```python
from build123d import *

# Parameters (mm, degrees)
SKETCH1_W                 = 76.2
SKETCH1_H                 = 76.2
BOSS_EXTRUDE1_DEPTH       = 3.175
SKETCH2_W                 = 69.79412
SKETCH2_H                 = 69.79412
BOSS_EXTRUDE2_DEPTH       = 9.525
F_6_32_TAPPED_HOLE1_D     = 2.7051
CIRPATTERN1_COUNT         = 4
SKETCH14_R                = 3.175
CUT_EXTRUDE1_DEPTH        = 56.358016583
SKETCH15_W                = 50.74412
SKETCH15_H                = 26.95956
CUT_EXTRUDE2_DEPTH        = 9.525
FILLET1_R                 = 12.7
F_6_32_TAPPED_HOLE2_D     = 2.7051
F_6_32_TAPPED_HOLE2_DEPTH = 9.652
F_6_32_TAPPED_HOLE2_TIP   = 0.81269403
FILLET1_OF_MIRROR3_R      = 12.7
SKETCH21_W                = 76.2
SKETCH21_H                = 76.2
CUT_EXTRUDE3_DEPTH        = 3.175


with BuildPart() as part:
    # Sketch1 → Boss-Extrude1 (new body)
    with BuildSketch(Plane(origin=(0, 0, 0), x_dir=(1, 0, 0), z_dir=(0, 1, 0))):
        Rectangle(SKETCH1_W, SKETCH1_H)
    extrude(amount=BOSS_EXTRUDE1_DEPTH)

    # Sketch2 → Boss-Extrude2 (add)
    with BuildSketch(Plane(origin=(0, 3.175, 0), x_dir=(1, 0, 0), z_dir=(0, 1, 0))):
        Rectangle(SKETCH2_W, SKETCH2_H)
    extrude(amount=BOSS_EXTRUDE2_DEPTH)

    # Sketch9 → #6-32 Tapped Hole3 (revolve, cut)
    with BuildSketch(Plane(origin=(34.89706, 7.9375, 12.7), x_dir=(0, 0, -1), z_dir=(0, 1, 0))):
        Polygon((0, 0), (0, 11.98869403), (1.35255, 11.176), (1.35255, 0), align=None)
    f_6_32_tapped_hole3 = revolve(axis=Axis((41.24706, 7.9375, 12.7), (-1, 0, 0)), mode=Mode.SUBTRACT)

    # Mirror1: #6-32 Tapped Hole3 across plane
    add(f_6_32_tapped_hole3.mirror(Plane.XY), mode=Mode.SUBTRACT)

    # Mirror2: #6-32 Tapped Hole3 across plane
    add(f_6_32_tapped_hole3.mirror(Plane(origin=(0, 0, 0), x_dir=(0, 0, 1), z_dir=(1, 0, 0))), mode=Mode.SUBTRACT)

    # Mirror2 copy 1 sketch → Mirror2 copy 1 (revolve, cut)
    with BuildSketch(Plane(origin=(-34.89706, 7.9375, -12.7), x_dir=(0, 0, 1), z_dir=(0, 1, 0))):
        Polygon((0, 0), (0, 11.98869403), (1.35255, 11.176), (1.35255, 0), align=None)
    revolve(axis=Axis((-41.24706, 7.9375, -12.7), (1, 0, 0)), mode=Mode.SUBTRACT)

    # #6-32 Tapped Hole1 (through all)
    with Locations(Plane(origin=(0, 0, 0), x_dir=(-1, 0, 0), z_dir=(0, -1, 0))):
        with Locations((-32.5501, 32.5501)):
            f_6_32_tapped_hole1 = Hole(F_6_32_TAPPED_HOLE1_D / 2)

    # CirPattern1: #6-32 Tapped Hole1 ×4 about axis
    cirpattern1_axis = Axis((0, 0, 0), (0, 1, 0))
    for i in range(1, CIRPATTERN1_COUNT):
        add(f_6_32_tapped_hole1.rotate(cirpattern1_axis, i * 360 / CIRPATTERN1_COUNT), mode=Mode.SUBTRACT)

    # Sketch14 → Cut-Extrude1 (cut, through all)
    with BuildSketch(Plane.XZ):
        with Locations(Location((0, 0, 0), (0, 0, 270))):
            Circle(SKETCH14_R)
    extrude(amount=-CUT_EXTRUDE1_DEPTH, mode=Mode.SUBTRACT)

    # Sketch15 → Cut-Extrude2 (cut)
    with BuildSketch(Plane(origin=(0, 12.7, 0), x_dir=(1, 0, 0), z_dir=(0, 1, 0))):
        with Locations((0, -21.41728)):
            Rectangle(SKETCH15_W, SKETCH15_H)
    cut_extrude2 = extrude(amount=-CUT_EXTRUDE2_DEPTH, mode=Mode.SUBTRACT)

    # Fillet1
    # the kernel refuses this fillet: 12.7 mm, written as the material it adds along each edge
    with BuildSketch(Plane(origin=(25.37206, 12.7, 7.9375), x_dir=(0, 0, 1), z_dir=(0, -1, 0))) as fillet1_piece_1_section:
        with BuildLine():
            CenterArc((FILLET1_R, FILLET1_R), FILLET1_R, 180, 90)
            Line((0, FILLET1_R), (0, 0))
            Line((0, 0), (FILLET1_R, 0))
        make_face()
    fillet1_piece_1 = extrude(amount=9.525, mode=Mode.PRIVATE)
    fillet1_piece_1 = fillet1_piece_1 - Plane(origin=(22.423937315, 7.9375, 12.7), x_dir=(0, 0, -1), z_dir=(1, 0, 0)) * Cylinder(1.35255, 70, mode=Mode.PRIVATE)
    add(fillet1_piece_1)
    with BuildSketch(Plane(origin=(-25.37206, 12.7, 7.9375), x_dir=(1, 0, 0), z_dir=(0, -1, 0))) as fillet1_piece_2_section:
        with BuildLine():
            CenterArc((FILLET1_R, FILLET1_R), FILLET1_R, 180, 90)
            Line((0, FILLET1_R), (0, 0))
            Line((0, 0), (FILLET1_R, 0))
        make_face()
    fillet1_piece_2 = extrude(amount=9.525, mode=Mode.PRIVATE)
    fillet1_piece_2 = fillet1_piece_2 - Plane(origin=(-22.423935797, 7.9375, 12.7), x_dir=(0, 0, -1), z_dir=(-1, 0, 0)) * Cylinder(1.35255, 70, mode=Mode.PRIVATE)
    add(fillet1_piece_2)

    # #6-32 Tapped Hole2
    with Locations(Plane.XY.offset(7.9375)):
        with Locations((0, 7.9375)):
            Hole(F_6_32_TAPPED_HOLE2_D / 2, depth=F_6_32_TAPPED_HOLE2_DEPTH)
            with Locations((0, 0, -(F_6_32_TAPPED_HOLE2_DEPTH + F_6_32_TAPPED_HOLE2_TIP / 2))):  # 118° drill point
                Cone(0, F_6_32_TAPPED_HOLE2_D / 2, F_6_32_TAPPED_HOLE2_TIP, mode=Mode.SUBTRACT)

    # Mirror3: Cut-Extrude2 across plane
    add(cut_extrude2.mirror(Plane.XY), mode=Mode.SUBTRACT)

    # Fillet1 of Mirror3
    # the kernel refuses this fillet: 12.7 mm, written as the material it adds along each edge
    with BuildSketch(Plane(origin=(25.37206, 12.7, -7.9375), x_dir=(-1, 0, 0), z_dir=(0, -1, 0))) as fillet1_of_mirror3_piece_1_section:
        with BuildLine():
            CenterArc((FILLET1_OF_MIRROR3_R, FILLET1_OF_MIRROR3_R), FILLET1_OF_MIRROR3_R, 180, 90)
            Line((0, FILLET1_OF_MIRROR3_R), (0, 0))
            Line((0, 0), (FILLET1_OF_MIRROR3_R, 0))
        make_face()
    fillet1_of_mirror3_piece_1 = extrude(amount=9.525, mode=Mode.PRIVATE)
    fillet1_of_mirror3_piece_1 = fillet1_of_mirror3_piece_1 - Plane(origin=(22.423935797, 7.9375, -12.7), x_dir=(0, 0, 1), z_dir=(1, 0, 0)) * Cylinder(1.35255, 70, mode=Mode.PRIVATE)
    add(fillet1_of_mirror3_piece_1)
    with BuildSketch(Plane(origin=(-25.37206, 12.7, -7.9375), x_dir=(0, 0, -1), z_dir=(0, -1, 0))) as fillet1_of_mirror3_piece_2_section:
        with BuildLine():
            CenterArc((FILLET1_OF_MIRROR3_R, FILLET1_OF_MIRROR3_R), FILLET1_OF_MIRROR3_R, 180, 90)
            Line((0, FILLET1_OF_MIRROR3_R), (0, 0))
            Line((0, 0), (FILLET1_OF_MIRROR3_R, 0))
        make_face()
    fillet1_of_mirror3_piece_2 = extrude(amount=9.525, mode=Mode.PRIVATE)
    fillet1_of_mirror3_piece_2 = fillet1_of_mirror3_piece_2 - Plane(origin=(-22.423937315, 7.9375, -12.7), x_dir=(0, 0, 1), z_dir=(-1, 0, 0)) * Cylinder(1.35255, 70, mode=Mode.PRIVATE)
    add(fillet1_of_mirror3_piece_2)

    # Sketch21 → Cut-Extrude3 (cut)
    with BuildSketch(Plane.XZ):
        Rectangle(SKETCH21_W, SKETCH21_H)
    extrude(amount=-CUT_EXTRUDE3_DEPTH, mode=Mode.SUBTRACT)


solid = part.part
```
Work out the finished part from the listing and answer in its coordinate system (mm). A direction names the side the tool comes from. Give positions to 0.01 mm unless a question says otherwise; leave off trailing zeros. Order: outer loops, then holes, each group sorted by start corner. A loop starts at its lowest first (then second) coordinate and runs counter-clockwise, first axis right, second up.
1. Section B-B, the plane x = 0 is taken. Determine the outline of the cut face in (y, z) (1 decimal).
Result sheet:
outline: (3.2, -7.9) - (12.7, -7.9) - (12.7, -3.2) - (3.2, -3.2) - close; (3.2, 3.2) - (6.6, 3.2) - (6.6, 7.9) - (3.2, 7.9) - close; (9.3, 3.2) - (12.7, 3.2) - (12.7, 7.9) - (9.3, 7.9) - close
2. Section D-D, the plane z = -12.7 is taken. Determine the outline of the cut face in (x, y) (3 decimals), and give its area (3 significant figures).
Result sheet:
outline: (-34.897, 3.175) - (-22.586, 3.175) - (-22.586, 6.585) - (-34.897, 6.585) - close; (-34.897, 9.29) - (-22.586, 9.29) - (-22.586, 12.7) - (-34.897, 12.7) - close; (22.586, 3.175) - (34.897, 3.175) - (34.897, 6.585) - (22.586, 6.585) - close; (22.586, 9.29) - (34.897, 9.29) - (34.897, 12.7) - (22.586, 12.7) - close
area: 168 mm2
3. For faces 4 (the cylindrical face through (-1.29, 8.34, 5.37)), 5 (the flat face through (0, 8, -7.938)), 6 (the flat face through (-25.372, 8, 28)), determine the directions among +Z, -Z, +X, -X, +Y, -Y from which every point of the face is accessible in a straight line to the end or side of a thin tool.
Result sheet:
face 4: +Z
face 5: -Z, +Y, -Y
face 6: +Z, +Y, -Y
4. Each of these flat-tipped pins is pushed along its axis until it touches: P1, Ø3, axis at x = 0.5, y = 10.5, coming from the +Z side; P2, Ø5, axis at x = 14.5, y = 11.5, coming from the -Z side; P3, Ø2, axis at x = -32.55, z = 32.55, coming from the +Y side; P4, Ø1.6, axis at x = 0, y = 7.94, coming from the -Z side. Where does it stop, or does it pass through?
Result sheet:
P1: stops at z = 7.94
P2: stops at z = -8.7
P3: passes through
P4: stops at z = -7.94
5. Straight lines are drawn through the part: L1, parallel to X at y = 8.5, z = 22.5; L2, parallel to X at y = 4, z = -32; L3, parallel to Z at x = 0, y = 9.25 (1 decimal). For each, find the intervals that lie inside material, in ascending order.
Result sheet:
L1: x = -34.9 to -25.37, 25.37 to 34.9
L2: x = -34.9 to -33.79, -31.31 to -25.37, 25.37 to 31.31, 33.79 to 34.9
L3: z = -7.9 to -3.2
6. Section A-A, the plane z = 0 is taken. Determine the outline of the cut face in (x, y) (3 decimals).
Result sheet:
outline: (-34.897, 3.175) - (-3.175, 3.175) - (-3.175, 12.7) - (-34.897, 12.7) - close; (3.175, 3.175) - (34.897, 3.175) - (34.897, 12.7) - (3.175, 12.7) - close
7. Section C-C, the plane y = 10.5 is taken. Give the number of separate pieces and of enclosed holes in the cut face, and give its area (3 significant figures).
Result sheet:
separate pieces: 1
enclosed holes: 5
area: 2,220 mm2
8. The mould has two halves that part along Z. Classify faces 1 (the cylindrical face through (21.553, 9.063, 11.559)), 2 (the cylindrical face through (-32.26, 8, 31.23)), 3 (the flat face through (34.897, 8, 0)): released by +Z, released by -Z, zero draft, split by the parting line, or undercut.
Result sheet:
face 1: released by +Z
face 2: undercut
face 3: zero draft
